Input: part model. Units: mm. Frame: model coordinates. Face numbers are marked on the shaded views. Coordinates: 2 decimals unless noted, no trailing zeros. Write each loop counter-clockwise with the first axis right and the second up, starting at its lowest first coordinate (ties: lowest second). Pieces come first, ordered by that corner, then holes. Notation, with made-up numbers: M 28.5,27 L 71.5,27 A11 ccw 71.5,47 Z; hole C -16,-34.75 d7. An arc over 180 degrees is marked long. Use CSV: the item, a comma, the result in double quotes.
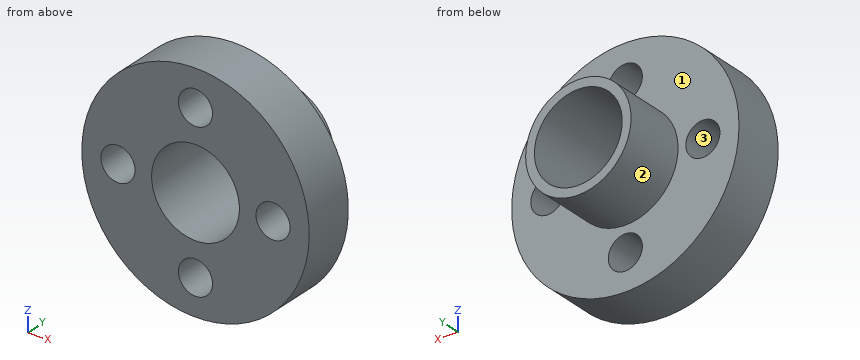
Autodesk Inventor part; units mm, degrees
ref_plane "YZ Plane" through (0, 0, 0) normal (1, 0, 0) x (0, 1, 0)
ref_plane "XZ Plane" through (0, 0, 0) normal (0, 1, 0) x (-1, 0, 0)
ref_plane "XY Plane" through (0, 0, 0) normal (0, 0, 1) x (1, 0, 0)
sketch "Sketch1" plane through (0, 0, 0) normal (0, 1, 0) x (-1, 0, 0)
  circle A0 centre (0, 0) radius 11
  circle A1 centre (0, 0) radius 4.25
  circle A2 centre (0, -7.5) radius 1.65
  circle A3 centre (7.5, 0) radius 1.65
  circle A4 centre (0, 7.5) radius 1.65
  circle A5 centre (-7.5, 0) radius 1.65
  dimension "d0" = 22
  dimension "d1" = 8.5
  dimension "d2" = 3.3
  dimension "d3" = 7.5
  dimension "d6" = 360
extrude "Extrusion1" add sketch "Sketch1" along normal blind 5
sketch "Sketch2" plane through (0, 5, 0) normal (0, 1, 0) x (1, 0, 0)
  circle A0 centre (0, 0) radius 4.25
  circle A1 centre (0, 0) radius 5.1
  dimension "d10" = 10.2
extrude "Extrusion2" add sketch "Sketch2" along normal blind 6
properties part number "ACOPLE_NUEVO_iMPOVISDO" material "Steel, Mild, Welded"
1. Section C-C (y = 3.5). Return loops of the section in (x, z), then the cut area to 3 significant figures.
Resolved:
outline,"C 0,0 d22; hole C -7.5,0 d3.3; hole C 0,0 d8.5; hole C 0,-7.5 d3.3; hole C 0,7.5 d3.3; hole C 7.5,0 d3.3"
area,"289 mm^2"
2. Section B-B (z = -8.25). Return loops of the section in (x, y).
Resolved:
outline,"M -7.28,0 L -1.47,0 L -1.47,5 L -7.28,5 Z; M 1.47,0 L 7.28,0 L 7.28,5 L 1.47,5 Z"
3. Mould query, pull axis X, two halves, no side actions, for the marked faces 1, 2 and 3. Classes: pulls with the +X half, pulls with the -X half, needs draft (parallel to the pull), parting line crosses it, or undercut.
Resolved:
face 1,"needs draft"
face 2,"parting line crosses it"
face 3,"undercut"
4. Section D-D (x = 6.75). Return loops of the section in (y, z), then the cut area to 3 significant figures.
Resolved:
outline,"M 0,-8.69 L 5,-8.69 L 5,-1.47 L 0,-1.47 Z; M 0,1.47 L 5,1.47 L 5,8.69 L 0,8.69 Z"
area,"72.2 mm^2"
5. Contact query for flat-ended pins moving along their axis: pin 1 Ø11 at (x, z) = (0, 0) entering from +Y; pin 2 Ø3 at (y, z) = (4, -8) entering from +X; pin 3 Ø4.5 at (x, z) = (7.5, 0) entering from +Y; pin 4 Ø1 at (x, y) = (8, 6.5) entering from +Z. Output: stop coordinate, or through.
Resolved:
pin 1,"stops at y = 11"
pin 2,"stops at x = 8.87"
pin 3,"stops at y = 5"
pin 4,"passes through"
6. Material intervals for line 1 (Z direction, x = 0, y = 3.7); line 2 (Y direction, x = -4.75, z = -9.75); line 3 (X direction, y = 2.5, z = 1.25), sorted ascending. Write a range as [from, to].
Resolved:
line 1,"z = [-11, -9.15], [-5.85, -4.25], [4.25, 5.85], [9.15, 11]"
line 2,"y = [0, 5]"
line 3,"x = [-10.93, -8.58], [-6.42, -4.06], [4.06, 6.42], [8.58, 10.93]"
